from build123d import *

# Parameters (mm, degrees)
F0_W     = 38.1
F0_H     = 50.8
F1_DEPTH = 6.35
F2_W     = 6.35
F2_H     = 6.910296
F3_DEPTH = 38.1
F6_W     = 50.8
F6_H     = 88.9
F7_DEPTH = 12.7


with BuildPart() as f1:
    # F0 (on Top) → F1 (new body)
    with BuildSketch(Plane.XY):
        Rectangle(F0_W, F0_H)
    extrude(amount=F1_DEPTH)

    # F2 (on face) → F3 (join)
    with BuildSketch(Plane.XY.offset(6.35)):
        Rectangle(F2_W, F2_H)
    extrude(amount=F3_DEPTH)

    # F6 (on face) → F7 (join)
    with BuildSketch(Plane(origin=(23.750519, 0, 19.929052), x_dir=(0, -1, 0), z_dir=(-0.766044, 0, -0.642788))):
        with Locations((0.969407, 78.143354)):
            Rectangle(F6_W, F6_H)
    extrude(amount=F7_DEPTH)


solid = f1.part
Geometry: final body of the model. Coordinates: model frame, mm. A direction names the side the tool comes from. Give positions to 0.01 mm unless a question says otherwise; leave off trailing zeros. Write each loop counter-clockwise with the first axis right and the second up, starting at its lowest first coordinate (ties: lowest second). Pieces come first, ordered by that corner, then holes. Notation, with made-up numbers: (13, 78) - (46, 78) arc R22 cw to (46, 103) - close; hole circle Ø3 at (16.5, 49). An arc over 180 degrees is marked (long way). Return JSON: item names as keys, results as strings. Group by question number.
1) Section B-B on y = -1.5. Return the cut outline in (x, z) (3 decimals), plus the area to 3 significant figures.
2) Section D-D on z = 30. Return the cut outline in (x, y) (3 decimals), plus the area to 3 significant figures.
3) First-contact query: P1, Ø2, axis at y = 1, z = 17, coming from the -X side (3 decimals); P2, Ø1, axis at x = -48, y = 11, coming from the +Z side; P3, Ø4, axis at y = 1.5, z = 72, coming from the -X side; P4, Ø3, axis at y = -20.5, z = 35, coming from the +X side. Flat tips, straight axial feed; report the tip coordinate or a pass-through.
4) Section A-A on y = -20.5. Return the cut outline in (x, z).
5) Mould query, pull axis Z, two halves, no side actions, for faces 4 (the flat face through (-36.608, -0.614, 72.104)), 5 (the flat face through (-59.847, -0.614, 109.816)), 6 (the flat face through (0, -25.4, 3)). Classes: released by +Z, released by -Z, zero draft, split by the parting line, or undercut.
6) Line query: line 1 (Y direction, x = -10, z = 56); line 2 (Y direction, x = 0.5, z = 18); line 3 (Z direction, x = 12, y = 4). Output: solid intervals per line, ascending.
7) Set-up query: faces 1 (the flat face through (0, 3.455, 25)), 2 (the flat face through (-19.05, 0, 3)), 3 (the flat face through (0, -3.455, 25)). Return all of +Z, -Z, +X, -X, +Y, -Y with unobstructed straight access to the full face (end or side cutting, diameter ignored); none if empty.
8) Section C-C on x = -9.5. Return the cut outline in (y, z).
Filled in:
{
 "1": {"outline": "(-64.78, 105.678) - (-7.636, 37.576) - (-3.175, 41.319) - (-3.175, 6.35) - (-19.05, 6.35) - (-19.05, 0) - (19.05, 0) - (19.05, 6.35) - (3.175, 6.35) - (3.175, 44.45) - (0.556, 44.45) - (2.093, 45.74) - (-55.051, 113.841) - close", "area": "1,610 mm^2"},
 "2": {"outline": "(-3.175, -3.455) - (3.175, -3.455) - (3.175, 3.455) - (-3.175, 3.455) - close", "area": "43.9 mm^2"},
 "3": {"P1": "stops at x = -3.175", "P2": "stops at z = 106.03", "P3": "stops at x = -38.2", "P4": "passes through"},
 "4": {"outline": "(-64.78, 105.68) - (-7.64, 37.58) - (2.09, 45.74) - (-55.05, 113.84) - close; (-19.05, 0) - (19.05, 0) - (19.05, 6.35) - (-19.05, 6.35) - close"},
 "5": {"face 4": "undercut", "face 5": "released by +Z", "face 6": "zero draft"},
 "6": {"line 1": "y = -26.37 to 24.43", "line 2": "y = -3.46 to 3.46", "line 3": "z = 0 to 6.35"},
 "7": {"face 1": "+X, +Y", "face 2": "-Z, -X, +Y, -Y", "face 3": "+X, -Y"},
 "8": {"outline": "(-26.37, 39.8) - (24.43, 39.8) - (24.43, 59.56) - (-26.37, 59.56) - close; (-25.4, 0) - (25.4, 0) - (25.4, 6.35) - (-25.4, 6.35) - close"}
}
